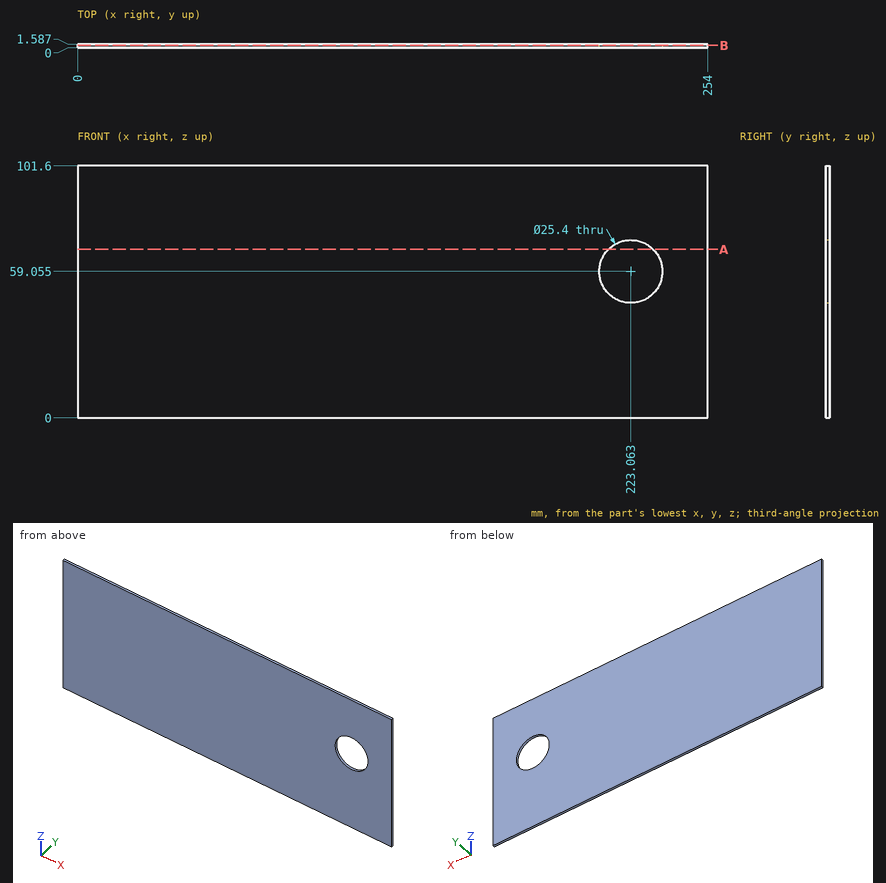
Source: three-view drawing plus pictorial views. Frame: mm from the lowest corner of the part. Round coordinates to 2 decimals unless told otherwise and drop trailing zeros. Order: outer loops, then holes, each group sorted by start corner. A loop starts at its lowest first (then second) coordinate and runs counter-clockwise, first axis right, second up. Notation, with made-up numbers: M -18.5,59.25 L -11.5,59.25 A15 ccw -11.5,81.25 Z; hole C 34.25,79.25 d4. An arc over 180 degrees is marked long. One line per item, written item: value.
(1) Cut plane B-B (y = 1). Return the cut outline in (x, z) (1 decimal).
Result sheet:
outline: M 0,0 L 254,0 L 254,101.6 L 0,101.6 Z; hole C 223.1,59.1 d25.4
(2) Cut plane A-A (z = 68). Return the cut outline in (x, y).
Result sheet:
outline: M 0,0 L 214.05,0 L 214.05,1.59 L 0,1.59 Z; M 232.08,0 L 254,0 L 254,1.59 L 232.08,1.59 Z
(3) Line query: probe 1 along X at (y, z) = (0.4, 62); probe 2 along X at (y, z) = (0.45, 51.5) (1 decimal). Output: solid intervals per line, ascending. Write a range as [from, to].
Result sheet:
probe 1: [0, 210.71], [235.42, 254]
probe 2: [0, 212.9], [233.3, 254]
(4) Pin query (flat end, axial travel): P1, Ø15, axis at x = 223.06, z = 59.05, coming from the -Y side (3 decimals). Return the tip coordinate at first contact, or that it passes through.
Result sheet:
P1: through
